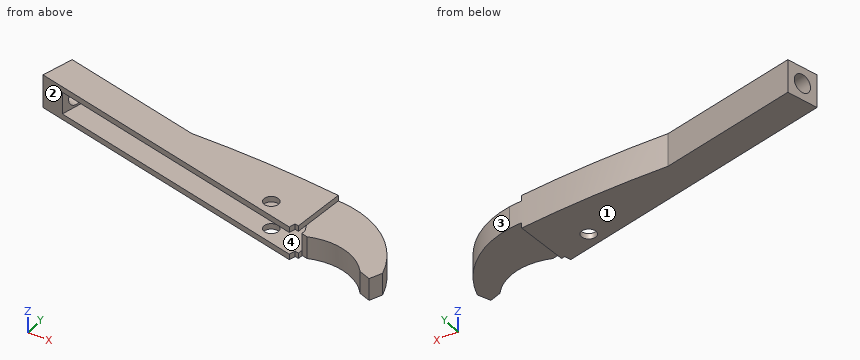
from build123d import *

# Parameters (mm, degrees)
SKETCH005_R     = 4
PAD003_DEPTH    = 9
POCKET002_DEPTH = 453.7991983662
POCKET003_DEPTH = 6
SKETCH009_R     = 5
POCKET004_DEPTH = 14


with BuildPart() as part:
    # Sketch005 → Pad003 (new body, symmetric)
    with BuildSketch(Plane.XY):
        with BuildLine():
            Line((129.191528, 8.290887), (132.069077, 15.263238))
            ThreePointArc((132.069077, 15.263238), (116.7747181113, 39.3905983189), (91.2212646928, 52.1604044318))
            ThreePointArc((91.2212646928, 52.1604044318), (46.3377236615, 57.1709115012), (1.21394, 59.036812))
            Line((-76.4001571445, 79.5700210048), (1.21394, 59.036812))
            Line((-76.4001571445, 79.5700210048), (-81.0037719697, 62.168678225))
            Line((-81.0037719697, 62.168678225), (78.772919, 19.898932))
            Line((78.772919, 19.898932), (79.701164, 23.416142))
            Line((79.701164, 23.416142), (87.415985, 21.315922))
            ThreePointArc((122.691841, 10.904919), (106.7527492861, 21.8666290226), (87.415985, 21.315922))
            Line((129.191528, 8.290887), (122.691841, 10.904919))
        make_face()
        with Locations((60.86446, 32.72789)):
            Circle(SKETCH005_R, mode=Mode.SUBTRACT)
    extrude(amount=PAD003_DEPTH, both=True)

    # Sketch007 → Pocket002 (cut, through all)
    with BuildSketch(Plane.XY.offset(6)):
        with BuildLine():
            Line((81.633926, 20.987476), (84.018715, 54.669346))
            Line((84.018715, 54.669346), (91.8155354317, 53.6254730737))
            ThreePointArc((133.5781814805, 14.8051820085), (118.8696341007, 40.855964108), (91.8155354317, 53.6254730737))
            Line((133.5781814805, 14.8051820085), (129.179794, 5.660023))
            Line((129.179794, 5.660023), (81.633926, 20.987476))
        make_face()
    pocket002 = extrude(amount=POCKET002_DEPTH, mode=Mode.SUBTRACT)

    # Mirrored: Pocket002 across XY
    add(pocket002.mirror(Plane.XY), mode=Mode.SUBTRACT)

    # Sketch008 → Pocket003 (cut, symmetric)
    with BuildSketch(Plane.XY):
        with BuildLine():
            Line((84.0540226162, 25.0066254975), (76.6128766006, 40.9426462345))
            ThreePointArc((76.6128766006, 40.9426462345), (71.2066025484, 47.6653428321), (63.3038481091, 51.1249556635))
            Line((63.3038481091, 51.1249556635), (2.088246, 55.768429))
            Line((2.088246, 55.768429), (-65.343964, 72.03257))
            Line((-65.343964, 72.03257), (-69.729797, 53.758251))
            Line((-69.729797, 53.758251), (84.0540226162, 17.940607))
            Line((84.0540226162, 17.940607), (84.0540226162, 25.0066254975))
        make_face()
    extrude(amount=POCKET003_DEPTH, both=True, mode=Mode.SUBTRACT)

    # Sketch009 (on DatumPlane) → Pocket004 (cut)
    with BuildSketch(Plane(origin=(-76.4001571445, 79.5700210048, 0), x_dir=(-0.2557563792, -0.9667412655, 0), z_dir=(-0.9667412655, 0.2557563792, 0))):
        with Locations((9, 0)):
            Circle(SKETCH009_R)
    extrude(amount=-POCKET004_DEPTH, mode=Mode.SUBTRACT)


solid = part.part
Build history of the part. All positions in model axes, mm. Face numbers are marked on the shaded views. Round coordinates to 2 decimals unless told otherwise and drop trailing zeros. Write each loop counter-clockwise with the first axis right and the second up, starting at its lowest first coordinate (ties: lowest second). Pieces come first, ordered by that corner, then holes. Notation, with made-up numbers: (-12, 82.5) -> (39, 82.5) arc R12 ccw to (39, 101.5) -> close; hole circle Ø1 at (-26, 50). An arc over 180 degrees is marked (long way). Use one line per item in the form item = value.
Q1. Drop flat-ended pins along their axis: P1, Ø13.5, axis at x = 109.5, y = 42, coming from the -Z side; P2, Ø5, axis at x = 60.86, y = 32.73, coming from the +Z side; P3, Ø3, axis at x = -57.5, z = 0.5, coming from the -Y side; P4, Ø3, axis at y = 24, z = 0.5, coming from the -X side. Give the stop position or say it passes through.
Conclusion:
P1 = -6
P2 = through
P3 = 69.78
P4 = 83.82
Q2. Band-saw the part on C-C, the plane x = 47. Write the cut outline in (y, z), then the cut area to 3 significant figures.
Conclusion:
outline = (28.3, -9) -> (57.12, -9) -> (57.12, 9) -> (28.3, 9) -> (28.3, 6) -> (52.36, 6) -> (52.36, -6) -> (28.3, -6) -> close
area = 230 mm²
Q3. Drill centre lines: L1, parallel to Z at x = -13, y = 44.5; L2, parallel to Z at x = 87.5, y = 36.5; L3, parallel to Y at x = -26, z = 7.5. Where is each one in solid material? Low to high.
Conclusion:
L1 = -9 to -6, 6 to 9
L2 = -6 to 6
L3 = 47.62 to 66.24
Q4. Band-saw the part on D-D, the plane x = 114. Write the cut outline in (y, z), then the cut area to 3 significant figures.
Conclusion:
outline = (18.68, -6) -> (41.73, -6) -> (41.73, 6) -> (18.68, 6) -> close
area = 277 mm²
Q5. Band-saw the part on A-A, the plane x = -39.5. Write the cut outline in (y, z).
Conclusion:
outline = (51.19, -9) -> (69.81, -9) -> (69.81, 9) -> (51.19, 9) -> (51.19, 6) -> (65.8, 6) -> (65.8, -6) -> (51.19, -6) -> close
Q6. Band-saw the part on B-B, the plane y = 47.5. Write the cut outline in (x, z).
Conclusion:
outline = (-25.56, -9) -> (83.51, -9) -> (83.51, -6) -> (104.91, -6) -> (104.91, 6) -> (83.51, 6) -> (83.51, 9) -> (-25.56, 9) -> (-25.56, 6) -> (71.42, 6) -> (71.42, -6) -> (-25.56, -6) -> close
Q7. Two-plate mould, pull along X, no slides. Class the marked faces 1, 2, 3 and 4: released by +X, released by -X, zero draft, split by the parting line, or undercut.
Conclusion:
face_1 = zero draft
face_2 = released by -X
face_3 = released by +X
face_4 = undercut
